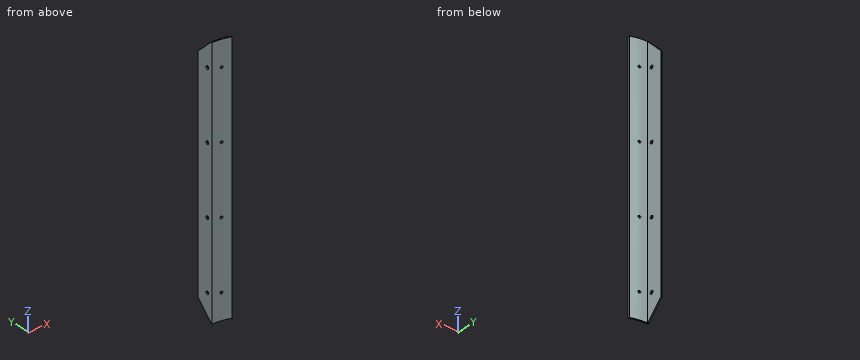
from build123d import *

# Parameters (mm, degrees)
EXTRUDE1_DEPTH               = 190.5
EXTRUDE2_DEPTH               = 387.35
F_6_CLEARANCE_HOLE1_D        = 3.6576
F_10_0_1935_DIAMETER_HOLE1_D = 4.9149
LPATTERN1_COUNT              = 3
LPATTERN1_PITCH              = 101.6
LPATTERN1_COL_COUNT          = 2
LPATTERN1_COL_PITCH          = 101.6


with BuildPart() as part:
    # Sketch1 → Extrude1 (new, symmetric)
    with BuildSketch(Plane.XY):
        with BuildLine():
            Line((0, 0), (0, 25.4))
            Line((0, 25.4), (1.5875, 25.4))
            Line((1.5875, 25.4), (1.5875, 1.5875))
            ThreePointArc((1.5875, 1.5875), (13.671867582, 0.546246178), (25.4, -2.546820159))
            Line((25.4, -2.546820159), (25.4, -4.781862636))
            ThreePointArc((25.4, -4.781862636), (12.923101507, -1.205874633), (0, 0))
        make_face()
    extrude(amount=EXTRUDE1_DEPTH, both=True)

    # Sketch2 → Extrude2 (cut)
    with BuildSketch(Plane.ZY):
        Polygon((190.5, 25.4), (166.6875, 25.4), (190.5, 1.5875), align=None)
    extrude2 = extrude(amount=-EXTRUDE2_DEPTH, mode=Mode.SUBTRACT)

    # Mirror2: Extrude2 across plane
    add(extrude2.mirror(Plane(origin=(0, 0, 0), x_dir=(1, 0, 0), z_dir=(0, 0, -1))), mode=Mode.SUBTRACT)

    # #6 Clearance Hole1 (through all)
    with Locations(Plane(origin=(0, 1.5875, 0), x_dir=(-1, 0, 0), z_dir=(0, 1, 0))):
        with Locations((-13.0175, -50.8)):
            f_6_clearance_hole1 = Hole(F_6_CLEARANCE_HOLE1_D / 2)

    # #10 (0.1935) Diameter Hole1 (through all)
    with Locations(Plane(origin=(1.5875, 8.5725, -50.8), x_dir=(0, 1, 0), z_dir=(1, 0, 0))):
        with Locations((0, 0)):
            f_10_0_1935_diameter_hole1 = Hole(F_10_0_1935_DIAMETER_HOLE1_D / 2)

    # LPattern1: #6 Clearance Hole1, #10 (0.1935) Diameter Hole1 ×3
    with Locations(*[(0, 0, i * LPATTERN1_PITCH) for i in range(1, LPATTERN1_COUNT)]):
        add(f_6_clearance_hole1, mode=Mode.SUBTRACT)
        add(f_10_0_1935_diameter_hole1, mode=Mode.SUBTRACT)

    # LPattern1 col: #6 Clearance Hole1, #10 (0.1935) Diameter Hole1 ×2
    with Locations(*[(0, 0, -i * LPATTERN1_COL_PITCH) for i in range(1, LPATTERN1_COL_COUNT)]):
        add(f_6_clearance_hole1, mode=Mode.SUBTRACT)
        add(f_10_0_1935_diameter_hole1, mode=Mode.SUBTRACT)


solid = part.part
CAD build for the part. Positions are in the model's coordinates, mm. Coordinates: 2 decimals unless noted, no trailing zeros. Loops run counter-clockwise (first coordinate to the right, second up) from the corner with the lowest first, then second, coordinate; pieces in that order, holes last. Notation, with made-up numbers: (-15, 4.5) - (35, 4.5) arc R35 cw to (35, 37.5) - close; hole circle Ø1 at (72, 33.25). An arc over 180 degrees is marked (long way). Use one line per item in the form item = value. Start each with the question number.
1) Drill centre lines: L1, parallel to X at y = 14.5, z = -86.5; L2, parallel to Y at x = 19.25, z = -70.5; L3, parallel to Y at x = 19.75, z = 87.5. Where is each one in solid material? Low to high. Write a range as from..to.
2) Flat gauge pins, fed straight in: pin 1 (5 mm diameter, centred on x = 13.02, z = -152.4, fed in from +Y); pin 2 (8 mm diameter, centred on x = 4.5, z = -53, fed in from +Y); pin 3 (10 mm diameter, centred on x = 13.5, z = 40, fed in from -Y); pin 4 (3 mm diameter, centred on x = 18, z = 10, fed in from -Y). Where does each tip first touch, or does it go through?
3) Band-saw the part on A-A (z = -64.5). Give the cut face in (x, y).
4) Band-saw the part on C-C (x = 7.25). Give the cut face in (y, z).
5) Band-saw the part on B-B (y = 19). Give the cut face in (x, z), and give its area (3 significant figures).
Check values:
q1.L1 = 0..1.59
q1.L2 = -2.7..-0.66
q1.L3 = -2.85..-0.79
q2.pin_1 = 1.02
q2.pin_2 = 25.4
q2.pin_3 = -2.49
q2.pin_4 = -2.78
q3.outline = (0, 0) arc R69.85 cw to (25.4, -4.78) - (25.4, -2.55) arc R70.64 ccw to (1.59, 1.59) - (1.59, 25.4) - (0, 25.4) - close
q4.outline = (-0.38, -190.5) - (1.36, -190.5) - (1.36, 190.5) - (-0.38, 190.5) - close
q5.outline = (0, -173.09) - (1.59, -173.09) - (1.59, 173.09) - (0, 173.09) - close
q5.area = 550 mm2
